from build123d import *

# Parameters (mm, degrees)
SKETCH1_W = 40
SKETCH1_H = 5
SKETCH2_W = 3.5
SKETCH2_H = 6


with BuildPart() as part:
    # Sketch1 → Base-Revolve (revolve)
    with BuildSketch(Plane.XY, mode=Mode.PRIVATE) as base_revolve_sk:
        with Locations((0, 2.5)):
            Rectangle(SKETCH1_W, SKETCH1_H)
    revolve(base_revolve_sk.sketch.rotate(Axis((-30, 0, 0), (1, 0, 0)), 90), axis=Axis((-30, 0, 0), (1, 0, 0)))

    # Sketch2 → Cut-to-GripLength (revolve, cut)
    with BuildSketch(Plane.XY):
        with Locations((-19.25, 3)):
            Rectangle(SKETCH2_W, SKETCH2_H)
        with Locations((19.25, 3)):
            Rectangle(SKETCH2_W, SKETCH2_H)
    revolve(axis=Axis((-30, 0, 0), (1, 0, 0)), mode=Mode.SUBTRACT)

    # Sketch3 → HeadTypeA (revolve)
    with BuildSketch(Plane.XY, mode=Mode.PRIVATE) as headtypea_sk:
        Polygon((-20, 5), (-20, 0), (-17.5, 0), (-17.5, 6.25), align=None)
        Polygon((20, 5), (17.5, 6.25), (17.5, 0), (20, 0), align=None)
    revolve(headtypea_sk.sketch.rotate(Axis((-23, 0, 0), (1, 0, 0)), 90), axis=Axis((-23, 0, 0), (1, 0, 0)))

    # Sketch5 → HoleTypeA (revolve, cut)
    with BuildSketch(Plane.XY, mode=Mode.PRIVATE) as holetypea_sk:
        Polygon((-12.690598923, 0), (-15, 4), (-20, 4), (-20, 0), align=None)
        Polygon((12.690598923, 0), (15, 4), (20, 4), (20, 0), align=None)
    revolve(holetypea_sk.sketch.rotate(Axis((-22, 0, 0), (1, 0, 0)), 90), axis=Axis((-22, 0, 0), (1, 0, 0)), mode=Mode.SUBTRACT)


solid = part.part
Design review of the part built by this model. Coordinates are the model's own, in mm. A direction names the side the tool comes from. Coordinates: 2 decimals unless noted, no trailing zeros. Loops run counter-clockwise (first coordinate to the right, second up) from the corner with the lowest first, then second, coordinate; pieces in that order, holes last. Notation, with made-up numbers: (59, 65) -> (111, 65) arc R24 cw to (111, 90) -> close; hole circle Ø3 at (-25, 20). An arc over 180 degrees is marked (long way). Use a Markdown table: item, result. Add a question column.
Item 1: Machinability: for faces 1 (the cylindrical face through (17.535, 3.905, -0.867)), 2 (the flat face through (17.5, -5, 2)), which of the approach directions +Z, -Z, +X, -X, +Y, -Y give a long, thin tool a straight path to every point of the face, cutting with its end or side? Answer none if there is none.
Item 2: Clearance check with flat-ended pins moving along their axes: P1, Ø6.5, axis at y = 0, z = 0, coming from the -X side; P2, Ø1.5, axis at x = 1.5, z = -4, coming from the -Y side; P3, Ø1, axis at x = 1, y = 2, coming from the +Z side. State where each tip first meets the part, or that it passes through.
Item 3: Wall thickness on L1, parallel to Y at x = 16.2, z = 0; L2, parallel to Y at x = 0, z = -3; L3, parallel to Z at x = 18, y = -3: over which ranges is each line inside the solid? List them lowest first. Write a range as from..to.
Item 4: We need section A-A, the plane x = -17. Write out the cut boundary in (y, z), and give its area (3 significant figures).
Item 5: The part is to be moulded in two halves that separate along X. For faces 3 (the flat face through (-17.5, -5, -2)), 4 (the conical face through (-13.092, 0.678, -0.151)), 5 (the cylindrical face through (-17.535, 3.905, -0.867)), say which applies: +X half, -X half, draft (parallel to the pull), parting line (faces both ways), or undercut.
Numbers:
| question | item | result |
|---|---|---|
| 1 | face 1 | +X |
| 1 | face 2 | none |
| 2 | P1 | stops at x = -14.57 |
| 2 | P2 | stops at y = -3.8 |
| 2 | P3 | stops at z = 4.77 |
| 3 | L1 | y = -5..-4, 4..5 |
| 3 | L2 | y = -4..4 |
| 3 | L3 | z = -5.2..-2.65, 2.65..5.2 |
| 4 | outline | circle Ø10 at (0, 0); hole circle Ø8 at (0, 0) |
| 4 | area | 28.3 mm^2 |
| 5 | face 3 | undercut |
| 5 | face 4 | -X half |
| 5 | face 5 | draft |
